Geometry: final body of the model. Coordinates: model frame, mm. Face numbers are marked on the shaded views. A direction names the side the tool comes from. Give positions to 0.01 mm unless a question says otherwise; leave off trailing zeros. Write each loop counter-clockwise with the first axis right and the second up, starting at its lowest first coordinate (ties: lowest second). Pieces come first, ordered by that corner, then holes.
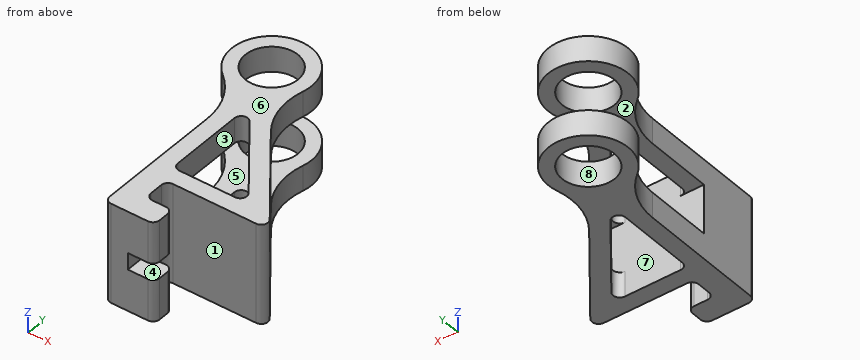
from build123d import *

# Parameters (mm, degrees)
BOSS_EXTRUDE1_DEPTH = 38.1
SKETCH2_R           = 15.24
BOSS_EXTRUDE2_DEPTH = 38.1
SKETCH3_R           = 10.033
SKETCH3_W           = 10.16
SKETCH3_H           = 10.16
CUT_EXTRUDE1_DEPTH  = 109.091847981
FILLET9_R           = 25.4
FILLET14_R          = 2.54
FILLET15_R          = 2.54
FILLET16_R          = 2.54
FILLET17_R          = 2.54
CUT_EXTRUDE2_REACH  = 124.665
SKETCH4_W           = 10.16
SKETCH4_H           = 6.35
SKETCH6_W           = 76.2
SKETCH6_H           = 18.796
CUT_EXTRUDE3_DEPTH  = 104.55757867


with BuildPart() as part:
    # Sketch1 → Boss-Extrude1 (new body)
    with BuildSketch(Plane(origin=(0, 0, 0), x_dir=(0, 1, 0), z_dir=(0, 0, 1))):
        Polygon((0, 48.26), (63.5, 48.26), (0, 0), (0, 29.21), (-19.05, 29.21), (-19.05, 48.26), align=None)
    extrude(amount=BOSS_EXTRUDE1_DEPTH)

    # Sketch2 → Boss-Extrude2 (add)
    with BuildSketch(Plane(origin=(0, 0, 38.1), x_dir=(0, -1, 0), z_dir=(0, 0, 1))):
        with Locations((-63.5, -48.26)):
            Circle(SKETCH2_R)
    extrude(amount=-BOSS_EXTRUDE2_DEPTH)

    # Sketch3 → Cut-Extrude1 (cut, through all)
    with BuildSketch(Plane.XY.offset(38.1)):
        with Locations((-48.26, 63.5)):
            Circle(SKETCH3_R)
        with Locations((-34.29, -5.08)):
            Rectangle(SKETCH3_W, SKETCH3_H)
        Polygon((-12.954, 6.35), (-41.91, 6.35), (-41.91, 44.45), align=None)
    extrude(amount=-CUT_EXTRUDE1_DEPTH, mode=Mode.SUBTRACT)

    # Fillet9
    fillet9_edges = [part.edges().sort_by_distance(p)[0] for p in [
        (-39.038531003, 51.366488162, 19.05),
        (-48.26, 48.26, 19.05),
    ]]
    fillet(fillet9_edges, radius=FILLET9_R)

    # Fillet14
    fillet14_edges = [part.edges().sort_by_distance(p)[0] for p in [
        (-41.91, 44.45, 19.05),
        (-12.954, 6.35, 19.05),
        (-41.91, 6.35, 19.05),
    ]]
    fillet(fillet14_edges, radius=FILLET14_R)

    # Fillet15
    fillet15_edges = [part.edges().sort_by_distance(p)[0] for p in [
        (-39.37, -10.16, 19.05),
        (-39.37, 0, 19.05),
    ]]
    fillet(fillet15_edges, radius=FILLET15_R)

    # Fillet16
    fillet16_edges = [part.edges().sort_by_distance(p)[0] for p in [
        (-29.21, -10.16, 19.05),
    ]]
    fillet(fillet16_edges, radius=FILLET16_R)

    # Fillet17
    fillet17_edges = [part.edges().sort_by_distance(p)[0] for p in [
        (-29.21, -19.05, 19.05),
        (-48.26, -19.05, 19.05),
        (0, 0, 19.05),
    ]]
    fillet(fillet17_edges, radius=FILLET17_R)

    # Sketch4 → Cut-Extrude2 (cut, up to next)
    with BuildSketch(Plane.XZ.offset(19.05), mode=Mode.PRIVATE) as cut_extrude2_sk1:
        with Locations((-34.29, 19.05)):
            Rectangle(SKETCH4_W, SKETCH4_H)
    cut_extrude2_tool1 = extrude(cut_extrude2_sk1.sketch, amount=-CUT_EXTRUDE2_REACH, mode=Mode.PRIVATE) & part.part
    add(cut_extrude2_tool1.solids().sort_by_distance((-34.29, -19.05, 19.05))[0], mode=Mode.SUBTRACT)

    # Sketch6 → Cut-Extrude3 (cut, through all)
    with BuildSketch(Plane(origin=(0, 6.35, 0), x_dir=(-1, 0, 0), z_dir=(0, 1, 0))):
        with Locations((27.795452673, 19.05)):
            Rectangle(SKETCH6_W, SKETCH6_H)
    extrude(amount=CUT_EXTRUDE3_DEPTH, mode=Mode.SUBTRACT)


solid = part.part
Q1. Pull-direction query (Z, two-part tool) for the marked faces 5, 6, 7 and 8; classes: released by +Z, released by -Z, zero draft, split by the parting line, or undercut.
Filled sheet:
face 5: undercut
face 6: released by +Z
face 7: undercut
face 8: zero draft
Q2. Ray query, line 1 along Y through (x, z) = (-37, 23); line 2 along Z through (x, y) = (-39, 44); line 3 along X through (y, z) = (63, 34). Return the intervals inside material, ascending.
Filled sheet:
line 1: y = -19.05 to -10.15, -0.01 to 6.35
line 2: z = 0 to 9.65, 28.45 to 38.1
line 3: x = -63.49 to -58.28, -38.24 to -33.03
Q3. Access query for the marked faces 1, 2, 3 and 4. Directions: +Z, -Z, +X, -X, +Y, -Y. A direction counts if a zero-diameter tool reaches every point of the face in a straight line with its end or side. Return the directions, or none.
Filled sheet:
face 1: +Z, -Z, +X
face 2: +X, -X, +Y
face 3: +Z, -Z
face 4: +X, -Y
Q4. Pin query (flat end, axial travel): P1, Ø7.5, axis at y = 24, z = 35.5, coming from the +X side; P2, Ø8.5, axis at y = -7.5, z = 20.5, coming from the +X side; P3, Ø1.5, axis at y = 0.5, z = 9.5, coming from the -X side; P4, Ø3, axis at x = -33.5, y = 8, coming from the -Z side. Return the tip coordinate at first contact, or that it passes through.
Filled sheet:
P1: stops at x = -15.39
P2: stops at x = -29.58
P3: stops at x = -48.26
P4: passes through
Q5. Section B-B on z = 11. Output: boundary loops of the cut face in (x, y).
Filled sheet:
outline: (-48.26, -16.51) arc R2.54 ccw to (-45.72, -19.05) - (-31.75, -19.05) arc R2.54 ccw to (-29.21, -16.51) - (-29.21, -12.7) arc R2.54 ccw to (-31.75, -10.16) - (-36.83, -10.16) arc R2.54 cw to (-39.37, -7.62) - (-39.37, -2.54) arc R2.54 cw to (-36.83, 0) - (-5.12, 0) arc R2.54 ccw to (-3.1, 4.08) - (-4.83, 6.35) - (-48.26, 6.35) - close
Q6. Section D-D on z = 6.5. Output: boundary loops of the cut face in (x, y) (3 decimals), plus the area to 3 significant figures.
Filled sheet:
outline: (-57.785, 51.603) arc R25.4 cw to (-48.26, 31.775) - (-48.26, -16.51) arc R2.54 ccw to (-45.72, -19.05) - (-31.75, -19.05) arc R2.54 ccw to (-29.21, -16.51) - (-29.21, -12.7) arc R2.54 ccw to (-31.75, -10.16) - (-36.83, -10.16) arc R2.54 cw to (-39.37, -7.62) - (-39.37, -2.54) arc R2.54 cw to (-36.83, 0) - (-5.121, 0) arc R2.54 ccw to (-3.098, 4.077) - (-29.064, 38.242) arc R25.4 cw to (-33.478, 59.792) arc R15.24 ccw (long way) to start; hole circle Ø20.066 at (-48.26, 63.5); hole (-41.91, 8.89) arc R2.54 ccw to (-39.37, 6.35) - (-18.075, 6.35) arc R2.54 ccw to (-16.052, 10.427) - (-37.348, 38.447) arc R2.54 ccw to (-41.91, 36.91) - close
area: 1,660 mm2
Q7. Section C-C on y = 63.5. Output: boundary loops of the cut face in (x, z).
Filled sheet:
outline: (-63.5, 0) - (-58.29, 0) - (-58.29, 9.65) - (-63.5, 9.65) - close; (-63.5, 28.45) - (-58.29, 28.45) - (-58.29, 38.1) - (-63.5, 38.1) - close; (-38.23, 0) - (-33.02, 0) - (-33.02, 9.65) - (-38.23, 9.65) - close; (-38.23, 28.45) - (-33.02, 28.45) - (-33.02, 38.1) - (-38.23, 38.1) - close
Q8. Section A-A on x = -56. Output: boundary loops of the cut face in (y, z).
Filled sheet:
outline: (50.03, 0) - (57.12, 0) - (57.12, 9.65) - (50.03, 9.65) - close; (50.03, 28.45) - (57.12, 28.45) - (57.12, 38.1) - (50.03, 38.1) - close; (69.88, 0) - (76.63, 0) - (76.63, 9.65) - (69.88, 9.65) - close; (69.88, 28.45) - (76.63, 28.45) - (76.63, 38.1) - (69.88, 38.1) - close
